from build123d import *

# Parameters (mm, degrees)
SKETCH1_W               = 500
SKETCH1_H               = 890
BOSS_EXTRUDE1_DEPTH     = 50
SKETCH2_R               = 20
BOSS_EXTRUDE2_DEPTH     = 105
MIRROR2_COPY_1_SKETCH_R = 20
MIRROR2_COPY_1_DEPTH    = 105


with BuildPart() as part:
    # Sketch1 → Boss-Extrude1 (new body)
    with BuildSketch(Plane(origin=(0, 0, 0), x_dir=(1, 0, 0), z_dir=(0, 1, 0))):
        Rectangle(SKETCH1_W, SKETCH1_H)
    extrude(amount=BOSS_EXTRUDE1_DEPTH)

    # Sketch2 → Boss-Extrude2 (add)
    with BuildSketch(Plane(origin=(250, 0, 0), x_dir=(0, 0, -1), z_dir=(1, 0, 0))):
        with Locations((345, 24.274325974)):
            Circle(SKETCH2_R)
    boss_extrude2 = extrude(amount=BOSS_EXTRUDE2_DEPTH)

    # Mirror1: Boss-Extrude2 across plane
    add(boss_extrude2.mirror(Plane.XY))

    # Mirror2: Boss-Extrude2 across plane
    add(boss_extrude2.mirror(Plane(origin=(0, 0, 0), x_dir=(0, 0, 1), z_dir=(1, 0, 0))))

    # Mirror2 copy 1 sketch → Mirror2 copy 1 (add)
    with BuildSketch(Plane.ZY.offset(250)):
        with Locations((345, 24.274325974)):
            Circle(MIRROR2_COPY_1_SKETCH_R)
    extrude(amount=MIRROR2_COPY_1_DEPTH)


solid = part.part
Geometry check sheet. Reference: the model listing, model coordinates, mm. A direction names the side the tool comes from. Round coordinates to 2 decimals unless told otherwise and drop trailing zeros. Loops run counter-clockwise (first coordinate to the right, second up) from the corner with the lowest first, then second, coordinate; pieces in that order, holes last. Notation, with made-up numbers: (31.5, 74.5) -> (76.5, 74.5) arc R22 ccw to (76.5, 91.5) -> close; hole circle Ø8 at (52, 34.25). An arc over 180 degrees is marked (long way). Answer as a JSON object with one key per item and string values. Group by question number.
Item 1: Set-up check for faces 1 (the face through (301.765, 16.614, 363.475)), 2 (the face through (-301.765, 16.614, -363.475)), 3 (the face through (355, 25, 345)): record each of +Z, -Z, +X, -X, +Y, -Y from which the full face is reachable in a straight line by a thin tool's end or side.
Item 2: Cross-section at B-B, the plane x = -302.5. Record the cut outline in (y, z), plus the area to 3 significant figures.
Item 3: Depth check by flat-ended pin: pin 1 Ø1.5 at (y, z) = (11.5, 85.5) entering from -X; pin 2 Ø15 at (y, z) = (37, 134.5) entering from +X. Enter the tip coordinate at first touch or a pass-through.
Item 4: Thickness scan on line 1 along Z through (x, y) = (287.5, 24); line 2 along X through (y, z) = (4.5, -367); line 3 along Z through (x, y) = (-315.5, 10.5). Record the ranges inside material, lowest first.
Item 5: Cross-section at A-A, the plane z = -345. Record the cut outline in (x, y), plus the area to 3 significant figures.
Item 6: Cross-section at C-C, the plane z = 79. Record the cut outline in (x, y).
Determined:
{
 "1": {"face 1": "+X", "face 2": "-X", "face 3": "+Z, -Z, +X, +Y, -Y"},
 "2": {"outline": "circle Ø40 at (24.27, -345); circle Ø40 at (24.27, 345)", "area": "2,510 mm²"},
 "3": {"pin 1": "stops at x = -250", "pin 2": "stops at x = 250"},
 "4": {"line 1": "z = -365 to -325, 325 to 365", "line 2": "x = -250 to 250", "line 3": "z = -359.5 to -330.5, 330.5 to 359.5"},
 "5": {"outline": "(-355, 4.27) -> (-250, 4.27) -> (-250, 0) -> (250, 0) -> (250, 4.27) -> (355, 4.27) -> (355, 44.27) -> (250, 44.27) -> (250, 50) -> (-250, 50) -> (-250, 44.27) -> (-355, 44.27) -> close", "area": "33,400 mm²"},
 "6": {"outline": "(-250, 0) -> (250, 0) -> (250, 50) -> (-250, 50) -> close"}
}
